Can you work these out from the drawing? Everything is in mm from the part's minimum corner. Round coordinates to 2 decimals unless told otherwise and drop trailing zeros. Order: outer loops, then holes, each group sorted by start corner. A loop starts at its lowest first (then second) coordinate and runs counter-clockwise, first axis right, second up. Notation, with made-up numbers: M -16.5,57.25 L 40.5,57.25 A32 ccw 40.5,88.25 Z; hole C 51,79.25 d11. An arc over 180 degrees is marked long. Write each question's results on one line, items separated by ' | '. Start each with the question number.
1. Please list where these lines run through material, in increasing order: L1, parallel to X at y = 62, z = 1.75; L2, parallel to Y at x = 49, z = 5.25; L3, parallel to Y at x = 19.5, z = 3.5.
2. I'm going to push flat-ended pins straight in: pin 1 (2 mm diameter, centred on x = 91.5, z = 2, fed in from -Y); pin 2 (2.5 mm diameter, centred on x = 174, z = 3.5, fed in from -Y); pin 3 (1 mm diameter, centred on y = 35.5, z = 1, fed in from -X). Where does each tip first touch, or does it pass through?
3. Suppose I cut it at C-C on x = 21. Write out the boundary of the cut face in (y, z), and give its area (3 significant figures).
4. Suppose I cut it at A-A on y = 59.5. Write out the boundary of the cut face in (x, z), and give its area (3 significant figures).
5. Suppose I cut it at B-B on z = 5.25. Write out the boundary of the cut face in (x, y).
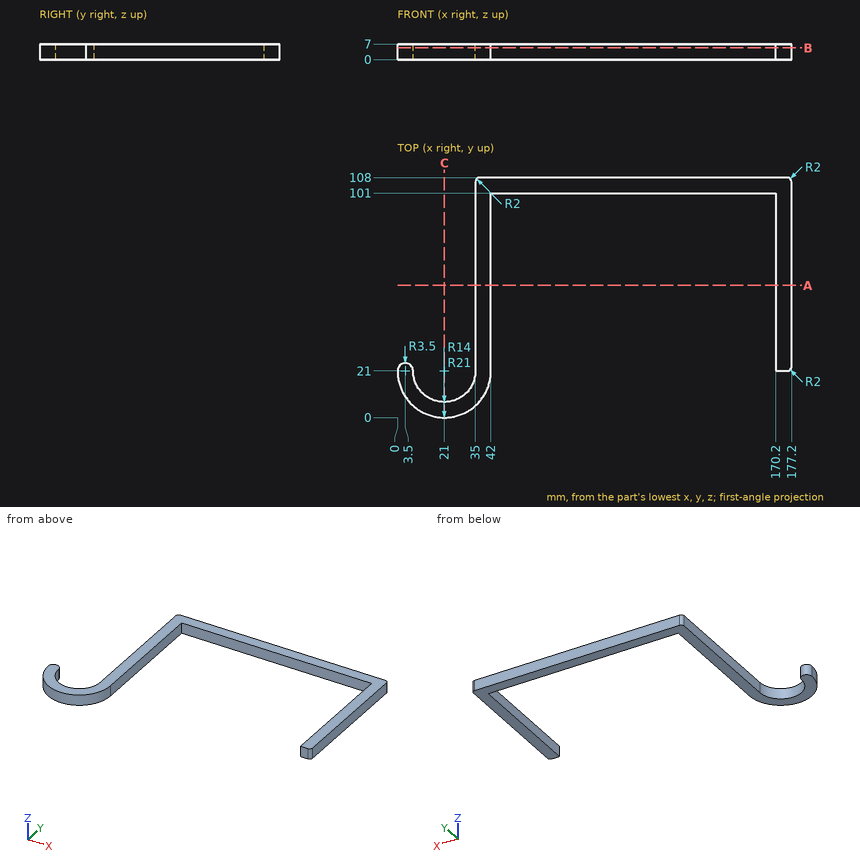
Filled sheet:
1) L1: x = 35 to 42, 170.2 to 177.2 | L2: y = 101 to 108 | L3: y = 0.05 to 7.08
2) pin 1: stops at y = 101 | pin 2: stops at y = 21 | pin 3: stops at x = 35
3) outline: M 0,0 L 7,0 L 7,7 L 0,7 Z | area: 49.0 mm^2
4) outline: M 35,0 L 42,0 L 42,7 L 35,7 Z; M 170.2,0 L 177.2,0 L 177.2,7 L 170.2,7 Z | area: 98.0 mm^2
5) outline: M 0,21 A21 ccw 42,21 L 42,101 L 170.2,101 L 170.2,21 L 175.2,21 A2 ccw 177.2,23 L 177.2,106 A2 ccw 175.2,108 L 37,108 A2 ccw 35,106 L 35,21 A14 cw 7,21 A3.5 ccw Z
